Read the model definition and answer for the solid it produces. Units are mm, in the model's axes. Face numbers are marked on the shaded views. A direction names the side the tool comes from. Coordinates: 2 decimals unless noted, no trailing zeros. Loops run counter-clockwise (first coordinate to the right, second up) from the corner with the lowest first, then second, coordinate; pieces in that order, holes last. Notation, with made-up numbers: (0.25, -29) -> (46.25, -29) arc R30 cw to (46.25, -2) -> close; hole circle Ø7 at (-39, 79.5). An arc over 180 degrees is marked (long way). Answer as a JSON object with one key per item and string values. Group by question number.
1) Section C-C, the plane y = 1.15 is taken. Give the vertices of the cut face in (x, z), plus the area to 3 significant figures.
2) Section B-B, the plane y = -1.8 is taken. Give the vertices of the cut face in (x, z).
3) A flat-ended cylindrical pin translates along its axis: P1, Ø3, axis at x = -22, z = -7.5, coming from the +Y side. Find the tip coordinate at first contact, or state that the pin passes through.
4) Consider probe 1 along Z at (x, y) = (2.5, -0.2); probe 2 along Z at (x, y) = (22, -1.85); probe 3 along X at (y, z) = (0.9, 2). Determine where each line is inside the solid, lowest interval first. Write a range as [from, to].
5) Which of the six approach directions +Z, -Z, +X, -X, +Y, -Y give full straight-line access (tool end or side, diameter ignored) to the marked faces 1 and 2?
6) Determine the mould class of the marked faces 3 and 4 for opening direction X: released by +X, released by -X, zero draft, split by the parting line, or undercut.
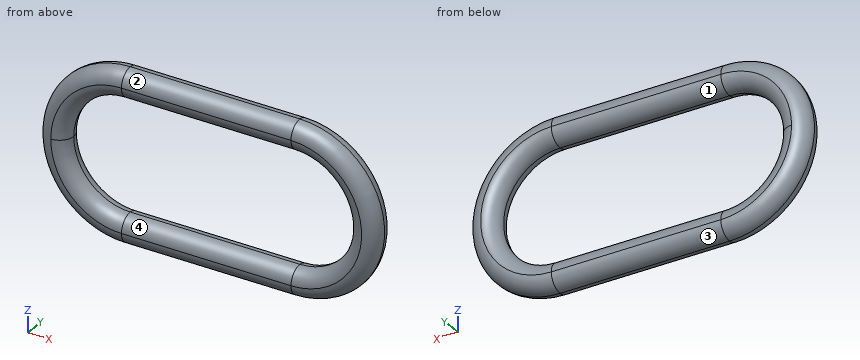
from build123d import *

# Parameters (mm, degrees)
F1_DEPTH      = 2.5
F1_DEPTH_BACK = 2.5
F2_R          = 2.49999


# Not quite as in the source:
# - a fillet or chamfer is up to 0.001 mm smaller than in the source, because OpenCascade refuses the exact size


with BuildPart() as f1:
    # F0 (on Front) → F1 (new body, two sides)
    with BuildSketch(Plane.XZ) as f1_sk:
        with BuildLine():
            ThreePointArc((15, -15), (25.6066017178, -10.6066017178), (30, 0))
            ThreePointArc((30, 0), (25.6066017178, 10.6066017178), (15, 15))
            Line((15, 15), (-15, 15))
            ThreePointArc((-15, 15), (-25.6066017178, 10.6066017178), (-30, 0))
            ThreePointArc((-30, 0), (-25.6066017178, -10.6066017178), (-15, -15))
            Line((-15, -15), (15, -15))
        make_face()
        with BuildLine():
            ThreePointArc((25, 0), (22.0710678119, -7.0710678119), (15, -10))
            Line((15, -10), (-15, -10))
            ThreePointArc((-15, -10), (-22.0710678119, -7.0710678119), (-25, 0))
            ThreePointArc((-25, 0), (-22.0710678119, 7.0710678119), (-15, 10))
            Line((-15, 10), (15, 10))
            ThreePointArc((15, 10), (22.0710678119, 7.0710678119), (25, 0))
        make_face(mode=Mode.SUBTRACT)
    extrude(amount=F1_DEPTH)
    extrude(f1_sk.sketch, amount=-F1_DEPTH_BACK)

    # F2 (radius 2.5 in the source; OpenCascade refuses exactly that, so slightly less here)
    f2_edges = [f1.edges().sort_by_distance(p)[0] for p in [
        (0, -2.5, -15),
        (0, 2.5, -15),
        (0, -2.5, -10),
        (0, 2.5, -10),
    ]]
    fillet(f2_edges, radius=F2_R)


solid = f1.part
Determined:
{
 "1": {"outline": "(-15, -14.72) -> (15, -14.72) arc R14.72 ccw to (15, 14.72) -> (-15, 14.72) arc R14.72 ccw to start; hole (-15, -10.28) -> (15, -10.28) arc R10.28 ccw to (15, 10.28) -> (-15, 10.28) arc R10.28 ccw to start", "area": "615 mm²"},
 "2": {"outline": "(-15, -14.23) -> (15, -14.23) arc R14.23 ccw to (15, 14.23) -> (-15, 14.23) arc R14.23 ccw to start; hole (-15, -10.77) -> (15, -10.77) arc R10.77 ccw to (15, 10.77) -> (-15, 10.77) arc R10.77 ccw to start"},
 "3": {"P1": "y = 2.39"},
 "4": {"probe 1": "[-14.99, -10.01], [10.01, 14.99]", "probe 2": "[-12.33, -8.25], [8.25, 12.33]", "probe 3": "[-29.7, -24.97], [24.97, 29.7]"},
 "5": {"face 1": "+Y", "face 2": "+Z, +X, -X, -Y"},
 "6": {"face 3": "zero draft", "face 4": "undercut"}
}
